```python
from build123d import *

# Parameters (mm, degrees)
SKETCH1_W            = 74
SKETCH1_H            = 59
EXTRUDE1_DEPTH       = 9
SKETCH2_R            = 5.5
CUT_EXTRUDE1_DEPTH   = 49.493093283
LPATTERN1_COUNT      = 2
LPATTERN1_PITCH      = 48
LPATTERN1_COUNT_DIR2 = 2
LPATTERN1_PITCH_DIR2 = 33
RIB2_START           = -9
RIB2_DEPTH           = 18
EXTRUDE2_DEPTH       = 9
SKETCH7_R            = 7.5
CUT_EXTRUDE2_DEPTH   = 9
FILLET8_R            = 13


# Read off the part's stored shape, not the designer's step: Rib2
with BuildPart() as part:
    # Sketch1 → Extrude1 (new body)
    with BuildSketch(Plane(origin=(0, 0, 0), x_dir=(1, 0, 0), z_dir=(0, 1, 0))):
        with Locations((0.345335821, 0.095708955)):
            Rectangle(SKETCH1_W, SKETCH1_H)
    extrude(amount=EXTRUDE1_DEPTH)

    # Sketch2 → Cut-Extrude1 (cut, through all)
    with BuildSketch(Plane(origin=(0, 9, 0), x_dir=(-1, 0, 0), z_dir=(0, 1, 0))):
        with Locations(Location((23.654664179, -16.595708955, 0), (0, 0, 90))):
            Circle(SKETCH2_R)
    cut_extrude1 = extrude(amount=-CUT_EXTRUDE1_DEPTH, mode=Mode.SUBTRACT)

    # LPattern1: Cut-Extrude1 2 × 2
    with Locations(*[(i * LPATTERN1_PITCH, 0, j * LPATTERN1_PITCH_DIR2) for i in range(LPATTERN1_COUNT) for j in range(LPATTERN1_COUNT_DIR2) if (i, j) != (0, 0)]):
        add(cut_extrude1, mode=Mode.SUBTRACT)

    # Rib2 outline → Rib2 (add)
    with BuildSketch(Plane(origin=(0.35, 0, 0), x_dir=(0, 0, -1), z_dir=(1, 0, 0)).offset(RIB2_START)):
        Polygon((29.595708955, 9), (-45.389590013, 81.412461489), (-64.138992076, 62.663059426), (-29.404291045, 0), (-29.404291045, 9), align=None)
    extrude(amount=RIB2_DEPTH)

    # Sketch6 → Extrude2 (add)
    with BuildSketch(Plane(origin=(0, 63.401025751, 63.401025751), x_dir=(1, 0, 0), z_dir=(0, 0.7071067811865438, 0.7071067811865513))):
        with BuildLine():
            Line((16.35, 27.956358014), (-15.65, 27.956358014))
            ThreePointArc((-15.65, 27.956358014), (-30.15, 13.456358014), (-15.65, -1.043641986))
            Line((-15.65, -1.043641986), (16.35, -1.043641986))
            ThreePointArc((16.35, -1.043641986), (30.85, 13.456358014), (16.35, 27.956358014))
        make_face()
    extrude(amount=EXTRUDE2_DEPTH)

    # Sketch7 → Cut-Extrude2 (cut)
    with BuildSketch(Plane(origin=(0, 69.764986782, 69.764986782), x_dir=(1, 0, 0), z_dir=(0, 0.7071067811865438, 0.7071067811865512))):
        with Locations(Location((16.35, 13.456358014, 0), (0, 0, 270))):
            Circle(SKETCH7_R)
        with Locations(Location((-15.65, 13.456358014, 0), (0, 0, 270))):
            Circle(SKETCH7_R)
    extrude(amount=-CUT_EXTRUDE2_DEPTH, mode=Mode.SUBTRACT)

    # Fillet8
    fillet8_edges = [part.edges().sort_by_distance(p)[0] for p in [
        (-36.654664179, 4.5, -29.595708955),
        (37.345335821, 4.5, -29.595708955),
        (37.345335821, 4.5, 29.404291045),
        (-36.654664179, 4.5, 29.404291045),
    ]]
    fillet(fillet8_edges, radius=FILLET8_R)


solid = part.part
```
Input: part model. Units: mm. Frame: model coordinates. A direction names the side the tool comes from. Round coordinates to 2 decimals unless told otherwise and drop trailing zeros. Write each loop counter-clockwise with the first axis right and the second up, starting at its lowest first coordinate (ties: lowest second). Pieces come first, ordered by that corner, then holes. Notation, with made-up numbers: (-19.5, 28) - (-5.5, 28) arc R23 cw to (-5.5, 57) - close; hole circle Ø4 at (6, 11.25). An arc over 180 degrees is marked (long way). Write item = value, one per line.
(1) Access query for faces 5 (the flat face through (-23, 9, -1)), 6 (the flat face through (23, 9, -1)), 7 (the flat face through (9.2, 72.9, 53.9)), 8 (the flat face through (17, 4, 29.404)), 9 (the flat face through (-16, 4, 29.404)). Directions: +Z, -Z, +X, -X, +Y, -Y. A direction counts if a zero-diameter tool reaches every point of the face in a straight line with its end or side. Return the directions, or none.
Geometry check:
face_5 = +Z, -Z, -X, +Y
face_6 = +Z, -Z, +X, +Y
face_7 = none
face_8 = +Z, +X, +Y, -Y
face_9 = +Z, -X, +Y, -Y
(2) Material intervals for probe 1 along X at (y, z) = (8.5, -18); probe 2 along X at (y, z) = (26.5, 12); probe 3 along Z at (x, y) = (-15, 5.5), sorted ascending.
Geometry check:
probe_1 = -36.58 to -28.97, -18.34 to 19.03, 29.66 to 37.27
probe_2 = -8.65 to 9.35
probe_3 = -29.6 to 29.4
(3) Section query D-D on x = -20.5. Output: boundary loops of the cut face in (y, z), then the cut area to 3 significant figures.
Geometry check:
outline = (0, -29.6) - (9, -29.6) - (9, -21.1) - (0, -21.1) - close; (0, -12.09) - (9, -12.09) - (9, 11.9) - (0, 11.9) - close; (0, 20.91) - (9, 20.91) - (9, 29.4) - (0, 29.4) - close; (63.25, 63.55) - (68.87, 57.93) - (75.23, 64.3) - (69.62, 69.91) - close; (76.96, 49.84) - (82.58, 44.22) - (88.94, 50.59) - (83.33, 56.2) - close
area = 512 mm^2
(4) Section query C-C on x = 4. Output: boundary loops of the cut face in (y, z).
Geometry check:
outline = (0, -29.6) - (9, -29.6) - (81.41, 45.39) - (83.17, 43.63) - (89.53, 50) - (69.03, 70.5) - (62.66, 64.14) - (0, 29.4) - close
(5) Contact query for flat-ended pins moving along their axis: pin 1 Ø3 at (y, z) = (66, 28) entering from -X; pin 2 Ø6 at (y, z) = (50.5, 57.5) entering from +X; pin 3 Ø7 at (x, y) = (19.5, 4.5) entering from +Z; pin 4 Ø6.5 at (x, z) = (-23.65, 16.4) entering from -Y. Output: stop coordinate, or through.
Geometry check:
pin_1 = -8.65
pin_2 = 9.35
pin_3 = 29.4
pin_4 = through
(6) Section query A-A on x = 11.5. Output: boundary loops of the cut face in (y, z).
Geometry check:
outline = (0, -29.6) - (9, -29.6) - (9, 29.4) - (0, 29.4) - close; (62.66, 64.14) - (68.87, 57.93) - (75.23, 64.3) - (69.03, 70.5) - close; (76.96, 49.84) - (83.17, 43.63) - (89.53, 50) - (83.33, 56.2) - close
(7) Pull-direction query (X, two-part tool) for faces 1 (the cylindrical face through (-28.534, 4.563, 18.942)), 2 (the cylindrical face through (22.239, 4.563, 21.485)), 3 (the flat face through (0, 4, -29.596)), 4 (the flat face through (-8.65, 41, 28)); classes: +X half, -X half, draft (parallel to the pull), parting line (faces both ways), or undercut.
Geometry check:
face_1 = undercut
face_2 = undercut
face_3 = draft
face_4 = -X half
(8) Section query B-B on z = -20. Output: boundary loops of the cut face in (x, y).
Geometry check:
outline = (-36.2, 0) - (-27.97, 0) - (-27.97, 9) - (-36.2, 9) - close; (-19.33, 0) - (20.03, 0) - (20.03, 9) - (9.35, 9) - (9.35, 18.27) - (-8.65, 18.27) - (-8.65, 9) - (-19.33, 9) - close; (28.67, 0) - (36.89, 0) - (36.89, 9) - (28.67, 9) - close
